For this review, take the finished solid that the model builds, in its own axes (mm). Give positions to 0.01 mm unless a question says otherwise; leave off trailing zeros. Write each loop counter-clockwise with the first axis right and the second up, starting at its lowest first coordinate (ties: lowest second). Pieces come first, ordered by that corner, then holes. Notation, with made-up numbers: (53, 40.25) -> (97, 40.25) arc R23 ccw to (97, 61.25) -> close; hole circle Ø4 at (-31.5, 42). An arc over 180 degrees is marked (long way). Return JSON: item names as keys, results as strings.
from build123d import *

# Parameters (mm, degrees)
CROQUIS1_R            = 7.25
BRIDA_BASE1_DEPTH     = 0.25
CROQUIS5_R            = 1.25
CORTAR_EXTRUIR1_DEPTH = 10
CORTAR_EXTRUIR2_DEPTH = 10


# Sheet-metal steps are written as plain solids
with BuildPart() as part:
    # Croquis1 → Brida base1 (new body)
    with BuildSketch(Plane.XY):
        Circle(CROQUIS1_R)
    extrude(amount=-BRIDA_BASE1_DEPTH)

    # Croquis5 → Cortar-Extruir1 (cut)
    with BuildSketch(Plane(origin=(0, 0, -0.25), x_dir=(-1, 0, 0), z_dir=(0, 0, -1))):
        Circle(CROQUIS5_R)
    extrude(amount=-CORTAR_EXTRUIR1_DEPTH, mode=Mode.SUBTRACT)

    # Croquis6 → Cortar-Extruir2 (cut)
    with BuildSketch(Plane.XY):
        Polygon((-5.480077554, 4.772970773), (-4.772970773, 5.480077554), (-4.494932198, 5.202038979), (-5.202038979, 4.494932198), align=None)
        Polygon((5.833630945, 4.419417382), (4.419417382, 5.833630945), (3.712310601, 5.126524164), (5.126524164, 3.712310601), align=None)
    extrude(amount=-CORTAR_EXTRUIR2_DEPTH, mode=Mode.SUBTRACT)


solid = part.part
1. Add section A-A, the plane x = 0. State the section outline as (y, z) points.
Results found:
{"outline": "(-7.25, -0.25) -> (-1.25, -0.25) -> (-1.25, 0) -> (-7.25, 0) -> close; (1.25, -0.25) -> (7.25, -0.25) -> (7.25, 0) -> (1.25, 0) -> close"}
2. Add section C-C, the plane z = -0.2. State the section outline as (x, y) points.
Results found:
{"outline": "(-5.47, 4.76) arc R7.25 ccw (long way) to (5.78, 4.37) -> (5.13, 3.71) -> (3.71, 5.13) -> (4.37, 5.78) arc R7.25 ccw to (-4.76, 5.47) -> (-4.49, 5.2) -> (-5.2, 4.49) -> close; hole circle Ø2.5 at (0, 0)"}
3. Add section D-D, the plane y = -4.25. State the section outline as (x, z) points, plus the area to 3 significant figures.
Results found:
{"outline": "(-5.87, -0.25) -> (5.87, -0.25) -> (5.87, 0) -> (-5.87, 0) -> close", "area": "2.94 mm²"}
4. To check wall thickness, follow probe 1 along Y at (x, z) = (0, -0.05); probe 2 along X at (y, z) = (-6.25, -0.1); probe 3 along X at (y, z) = (-3.25, -0.2). State the ranges of each line that lie inside material, in increasing order.
Results found:
{"probe 1": "y = -7.25 to -1.25, 1.25 to 7.25", "probe 2": "x = -3.67 to 3.67", "probe 3": "x = -6.48 to 6.48"}
